from build123d import *

# Parameters (mm, degrees)
SKETCH1_R                = 37.5
SKETCH1_R_2              = 20
BASE_FLANGE1_DEPTH       = 2.38125
BOSS_EXTRUDE1_DEPTH      = 2.38125
BOSS_EXTRUDE2_DEPTH      = 2.38125
FILLET1_R                = 3
CIRPATTERN1_COUNT        = 4
FILLET1_OF_CIRPATTERN1_R = 3
SKETCH7_R                = 0.5
CUT_EXTRUDE1_DEPTH       = 112.041300207
SKETCH10_R               = 0.79375
CUT_EXTRUDE2_DEPTH       = 112.041300207


# Sheet-metal steps are written as plain solids
with BuildPart() as part:
    # Sketch1 → Base-Flange1 (new body)
    with BuildSketch(Plane(origin=(0, 0, 0), x_dir=(1, 0, 0), z_dir=(0, 1, 0))):
        with Locations(Location((0, 0, 0), (0, 0, 270))):
            Circle(SKETCH1_R)
        with Locations(Location((0, 0, 0), (0, 0, 270))):
            Circle(SKETCH1_R_2, mode=Mode.SUBTRACT)
    extrude(amount=-BASE_FLANGE1_DEPTH)

    # Sketch6 → Boss-Extrude1 (add)
    with BuildSketch(Plane(origin=(0, 0, 0), x_dir=(1, 0, 0), z_dir=(0, 1, 0))):
        with BuildLine():
            Line((-3.5, 75), (-3.5, 37.336309405))
            Line((-3.5, 37.336309405), (3.5, 37.336309405))
            Line((3.5, 37.336309405), (3.5, 75))
            ThreePointArc((3.5, 75), (0, 78.5), (-3.5, 75))
        make_face()
    boss_extrude1 = extrude(amount=-BOSS_EXTRUDE1_DEPTH)

    # Sketch9 → Boss-Extrude2 (add)
    with BuildSketch(Plane(origin=(0, 0, 0), x_dir=(1, 0, 0), z_dir=(0, 1, 0))):
        with BuildLine():
            Line((23.925883831, 28.875631299), (28.875631299, 23.925883831))
            Line((28.875631299, 23.925883831), (44.901280605, 39.951533137))
            ThreePointArc((44.901280605, 39.951533137), (44.901280605, 44.901280605), (39.951533137, 44.901280605))
            Line((39.951533137, 44.901280605), (23.925883831, 28.875631299))
        make_face()
    boss_extrude2 = extrude(amount=-BOSS_EXTRUDE2_DEPTH)

    # Fillet1
    fillet1_edges = [part.edges().sort_by_distance(p)[0] for p in [
        (3.5, -1.190625, -37.336309405),
        (-3.5, -1.190625, -37.336309405),
        (23.925883831, -1.190625, -28.875631299),
        (28.875631299, -1.190625, -23.925883831),
    ]]
    fillet(fillet1_edges, radius=FILLET1_R)

    # CirPattern1: Boss-Extrude1, Boss-Extrude2 ×4 about axis
    cirpattern1_axis = Axis((0, 0, 0), (0, 1, 0))
    add([boss_extrude1.rotate(cirpattern1_axis, i * 360 / CIRPATTERN1_COUNT) for i in range(1, CIRPATTERN1_COUNT)])
    add([boss_extrude2.rotate(cirpattern1_axis, i * 360 / CIRPATTERN1_COUNT) for i in range(1, CIRPATTERN1_COUNT)])

    # Fillet1 of CirPattern1
    fillet1_of_cirpattern1_edges = [part.edges().sort_by_distance(p)[0] for p in [
        (-37.336309405, -1.190625, -3.5),
        (-37.336309405, -1.190625, 3.5),
        (-28.875631299, -1.190625, -23.925883831),
        (-23.925883831, -1.190625, -28.875631299),
        (-3.5, -1.190625, 37.336309405),
        (3.5, -1.190625, 37.336309405),
        (-23.925883831, -1.190625, 28.875631299),
        (-28.875631299, -1.190625, 23.925883831),
        (37.336309405, -1.190625, 3.5),
        (37.336309405, -1.190625, -3.5),
        (28.875631299, -1.190625, 23.925883831),
        (23.925883831, -1.190625, 28.875631299),
    ]]
    fillet(fillet1_of_cirpattern1_edges, radius=FILLET1_OF_CIRPATTERN1_R)

    # Sketch7 → Cut-Extrude1 (cut, through all)
    with BuildSketch(Plane(origin=(0, 0, 0), x_dir=(1, 0, 0), z_dir=(0, 1, 0))):
        with Locations(Location((-1.190625, 75, 0), (0, 0, 270))):
            Circle(SKETCH7_R)
        with Locations(Location((1.190625, 75, 0), (0, 0, 270))):
            Circle(SKETCH7_R)
        with Locations(Location((41.58450786, 43.268305883, 0), (0, 0, 270))):
            Circle(SKETCH7_R)
        with Locations(Location((43.268305883, 41.58450786, 0), (0, 0, 270))):
            Circle(SKETCH7_R)
        with Locations(Location((-75, -1.190625, 0), (0, 0, 270))):
            Circle(SKETCH7_R)
        with Locations(Location((-75, 1.190625, 0), (0, 0, 270))):
            Circle(SKETCH7_R)
        with Locations(Location((43.268305883, -41.58450786, 0), (0, 0, 270))):
            Circle(SKETCH7_R)
        with Locations(Location((41.58450786, -43.268305883, 0), (0, 0, 270))):
            Circle(SKETCH7_R)
    extrude(amount=-CUT_EXTRUDE1_DEPTH, mode=Mode.SUBTRACT)

    # Sketch10 → Cut-Extrude2 (cut, through all)
    with BuildSketch(Plane(origin=(0, 0, 0), x_dir=(1, 0, 0), z_dir=(0, 1, 0))):
        with Locations(Location((-23.573172318, 1.122532015, 0), (0, 0, 270))):
            Circle(SKETCH10_R)
        with Locations(Location((-1.122532015, 23.573172318, 0), (0, 0, 270))):
            Circle(SKETCH10_R)
        with Locations(Location((23.573172318, -1.122532015, 0), (0, 0, 270))):
            Circle(SKETCH10_R)
        with Locations(Location((1.122532015, -23.573172318, 0), (0, 0, 270))):
            Circle(SKETCH10_R)
    extrude(amount=-CUT_EXTRUDE2_DEPTH, mode=Mode.SUBTRACT)


solid = part.part
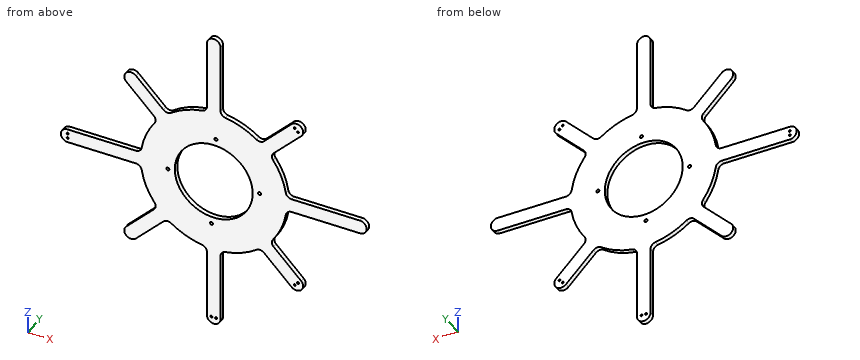
The model under review builds one solid part; all positions refer to its coordinate system, in mm. Coordinates: 2 decimals unless noted, no trailing zeros. Write each loop counter-clockwise with the first axis right and the second up, starting at its lowest first coordinate (ties: lowest second). Pieces come first, ordered by that corner, then holes. Notation, with made-up numbers: M -35,11 L 0,11 A17 ccw 0,31 Z; hole C -22,38.25 d6. An arc over 180 degrees is marked long. Put each result on its own line as item: value.
1) Add section B-B on x = 14.5. Give the boundary of the cut face in (y, z).
Computed:
outline: M -2.38,-34.58 L 0,-34.58 L 0,-13.77 L -2.38,-13.77 Z; M -2.38,13.77 L 0,13.77 L 0,34.58 L -2.38,34.58 Z
2) Clearance check with flat-ended pins moving along their axes: pin 1 Ø1.2 at (x, y) = (60.5, -0.5) entering from -Z; pin 2 Ø1 at (y, z) = (-0.5, -47) entering from +X; pin 3 Ø0.7 at (x, y) = (62, -1.5) entering from +Z. State where each tip first meets the part, or that it passes through.
Computed:
pin 1: stops at z = -3.5
pin 2: stops at x = 3.5
pin 3: stops at z = 3.5
3) Wall thickness on probe 1 along X at (y, z) = (-0.8, -75); probe 2 along X at (y, z) = (-0.05, 33); probe 3 along Z at (x, y) = (-38, -1.45): over which ranges is each line inside the solid? List them lowest first. Write a range as [from, to].
Computed:
probe 1: x = [-3.5, -1.69], [-0.69, 0.69], [1.69, 3.5]
probe 2: x = [-37.95, -28.05], [-17.81, 17.81], [28.05, 37.95]
probe 3: z = [-42.95, -33.05], [-4.24, 4.24], [33.05, 42.95]
4) Add section A-A on x = -9.5. Give the boundary of the cut face in (y, z), then the cut area to 3 significant figures.
Computed:
outline: M -2.38,-36.28 L 0,-36.28 L 0,-17.6 L -2.38,-17.6 Z; M -2.38,17.6 L 0,17.6 L 0,36.28 L -2.38,36.28 Z
area: 88.9 mm2
5) Add section C-C on y = -0.85. State how many separate pieces and enclosed holes the cut face has, then the cut area to 3 significant figures.
Computed:
separate pieces: 1
enclosed holes: 13
area: 5,010 mm2
